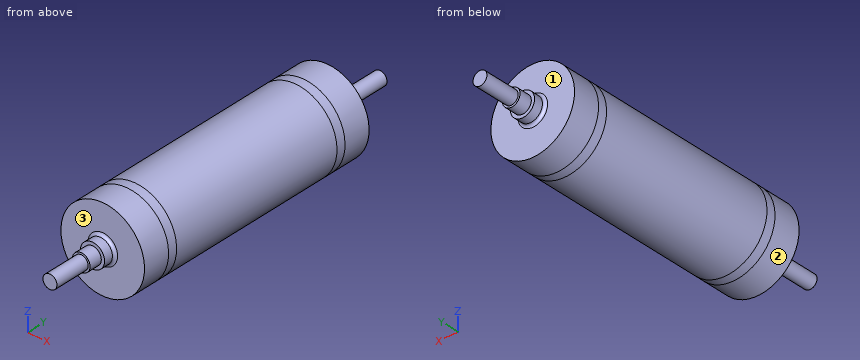
from build123d import *

# Parameters (mm, degrees)
F0_W = 195
F0_H = 37.5


with BuildPart() as f1:
    # F0 (on Right) → F1 (revolve)
    with BuildSketch(Plane.YZ):
        with BuildLine():
            ThreePointArc((15, 65), (4.393398, 69.393398), (0, 80))
            Line((0, 80), (0, 225))
            Line((0, 225), (-150, 225))
            Line((-150, 225), (-200, 224.925))
            Line((-200, 224.925), (-700, 224.925))
            Line((-700, 224.925), (-700, 0))
            Line((-700, 0), (0, 0))
            Line((0, 0), (64, 0))
            Line((64, 0), (64, 47.5))
            Line((64, 47.5), (64, 65))
            Line((64, 65), (15, 65))
        make_face()
        Polygon((134, 47.5), (64, 47.5), (64, 0), (134, 0), (134, 37.5), align=None)
        Polygon((-700, 0), (-700, 224.925), (-1200, 224.925), (-1250, 225), (-1400, 225), (-1400, 80), (-1400, 0), align=None)
        with Locations((231.5, 18.75)):
            Rectangle(F0_W, F0_H)
        with BuildLine():
            Line((-1464, 0), (-1400, 0))
            Line((-1400, 0), (-1400, 80))
            ThreePointArc((-1400, 80), (-1404.393398, 69.393398), (-1415, 65))
            Line((-1415, 65), (-1464, 65))
            Line((-1464, 65), (-1464, 47.5))
            Line((-1464, 47.5), (-1464, 0))
        make_face()
        Polygon((-1534, 0), (-1464, 0), (-1464, 47.5), (-1534, 47.5), (-1534, 37.5), align=None)
        with Locations((-1631.5, 18.75)):
            Rectangle(F0_W, F0_H)
    revolve(axis=Axis((0, -350, 0), (0, -1, 0)))


solid = f1.part
Geometry check sheet. Reference: the model listing, model coordinates, mm. Face numbers are marked on the shaded views. A direction names the side the tool comes from. Give positions to 0.01 mm unless a question says otherwise; leave off trailing zeros. Loops run counter-clockwise (first coordinate to the right, second up) from the corner with the lowest first, then second, coordinate; pieces in that order, holes last. Notation, with made-up numbers: (85.25, 77) -> (94.25, 77) arc R21 ccw to (94.25, 107) -> close; hole circle Ø3 at (11.5, -13). An arc over 180 degrees is marked (long way). Answer in a Markdown table with one row per item. Add a question column.
1) Gauge pin test, flat ends, axial feed: P1, Ø10, axis at x = -138.5, y = -413, coming from the -Z side; P2, Ø1.5, axis at x = -17.5, z = 46, coming from the +Y side; P3, Ø12, axis at x = 65.5, z = -142, coming from the -Y side. Record the tip position at first contact, or that the pin passes through.
2) Cross-section at A-A on y = -345.5. Record the boundary of the cut face in (x, z) (3 decimals).
3) Material ranges on probe 1 along Y at (x, z) = (-40, -7.5); probe 2 along Y at (x, z) = (57, -64); probe 3 along X at (y, z) = (-1494.5, 3.5), recorded low to high. Write a range as from..to.
4) Set-up check for the marked faces 1, 2 and 3: record each of +Z, -Z, +X, -X, +Y, -Y from which the full face is reachable in a straight line by a thin tool's end or side.
Outcome:
| question | item | result |
|---|---|---|
| 1 | P1 | stops at z = -181.02 |
| 1 | P2 | stops at y = 64 |
| 1 | P3 | stops at y = -1400 |
| 2 | outline | circle Ø449.85 at (0, 0) |
| 3 | probe 1 | y = -1534..134 |
| 3 | probe 2 | y = -1400..0 |
| 3 | probe 3 | x = -47.37..47.37 |
| 4 | face 1 | +Y |
| 4 | face 2 | +Y, -Y |
| 4 | face 3 | -Y |
